Here's how the part is built. I have some questions about the finished solid (model axes, mm). Face numbers are marked on the shaded views. A direction names the side the tool comes from. Coordinates: 2 decimals unless noted, no trailing zeros. Use one line per item in the form item = value. Start each with the question number.
from build123d import *

# Parameters (mm, degrees)
SCHIZZO1_W                     = 23
SCHIZZO1_H                     = 23
ESTRUSIONE_ESTRUSIONE1_DEPTH   = 50
SCHIZZO3_R                     = 17
TAGLIO_ESTRUSIONE2_DEPTH       = 58.057295879
SCHIZZO4_R                     = 17
SCHIZZO4_R_2                   = 15
ESTRUSIONE_ESTRUSIONE2_DEPTH   = 23
ESTRUSIONE_ESTRUSIONE3_START   = -2
SCHIZZO6_R                     = 15
ESTRUSIONE_ESTRUSIONE3_DEPTH   = 2
ESTRUSIONE_ESTRUSIONE4_START   = 1
SCHIZZO11_R                    = 15
ESTRUSIONE_ESTRUSIONE4_DEPTH   = 1
SMUSSO2_SIZE                   = 2
SCHIZZO12_R                    = 2.5
TAGLIO_ESTRUSIONE6_DEPTH       = 85.53268453
SCHIZZO13_R                    = 4.75
TAGLIO_ESTRUSIONE7_DEPTH       = 2
SCHIZZO14_R                    = 1.5
TAGLIO_ESTRUSIONE9_DEPTH       = 85.53268453
TAGLIO_ESTRUSIONE11_DEPTH      = 85.53268453
TAGLIO_ESTRUSIONE12_REACH      = 85.286
TAGLIO_ESTRUSIONE12_END_RADIUS = 15
SCHIZZO18_R                    = 7.1
ESTRUSIONE_ESTRUSIONE5_REACH   = 87.292
SCHIZZO19_W                    = 4
SCHIZZO19_H                    = 3
SCHIZZO21_R                    = 5.5
ESTRUSIONE_ESTRUSIONE6_DEPTH   = 2
SCHIZZO20_R                    = 1.75
TAGLIO_ESTRUSIONE13_DEPTH      = 86.853216328
SMUSSO3_SIZE                   = 2
SMUSSO4_SIZE                   = 1
SMUSSO4_SIZE2                  = 3


with BuildPart() as part:
    # Schizzo1 → Estrusione-Estrusione1 (new body)
    with BuildSketch(Plane.XY):
        with Locations((-3.551080126, 2.313028552)):
            Rectangle(SCHIZZO1_W, SCHIZZO1_H)
    extrude(amount=ESTRUSIONE_ESTRUSIONE1_DEPTH)

    # Schizzo3 → Taglio-Estrusione2 (cut, through all)
    with BuildSketch(Plane(origin=(0, 13.813028552, 0), x_dir=(1, 0, 0), z_dir=(0, 1, 0))):
        with Locations((-3.551080126, -62.519984026)):
            Circle(SCHIZZO3_R)
    extrude(amount=-TAGLIO_ESTRUSIONE2_DEPTH, mode=Mode.SUBTRACT)

    # Schizzo4 → Estrusione-Estrusione2 (add, through all)
    with BuildSketch(Plane(origin=(0, 13.813028552, 0), x_dir=(1, 0, 0), z_dir=(0, 1, 0))):
        with Locations((-3.551080126, -62.519984026)):
            Circle(SCHIZZO4_R)
        with Locations(Location((-3.551080126, -62.519984026, 0), (0, 0, 180))):
            Circle(SCHIZZO4_R_2, mode=Mode.SUBTRACT)
    extrude(amount=-ESTRUSIONE_ESTRUSIONE2_DEPTH)

    # Schizzo6 → Estrusione-Estrusione3 (add)
    with BuildSketch(Plane.XZ.offset(9.186971448).offset(ESTRUSIONE_ESTRUSIONE3_START)):
        with Locations(Location((-3.551080126, 62.519984026, 0), (0, 0, 180))):
            Circle(SCHIZZO6_R)
    extrude(amount=ESTRUSIONE_ESTRUSIONE3_DEPTH)

    # Schizzo11 → Estrusione-Estrusione4 (add)
    with BuildSketch(Plane(origin=(0, -7.186971448, 0), x_dir=(1, 0, 0), z_dir=(0, 1, 0)).offset(ESTRUSIONE_ESTRUSIONE4_START)):
        with Locations(Location((-3.551080126, -62.519984026, 0), (0, 0, 180))):
            Circle(SCHIZZO11_R)
    extrude(amount=-ESTRUSIONE_ESTRUSIONE4_DEPTH)

    # Smusso2
    smusso2_edges = [part.edges().sort_by_distance(p)[0] for p in [
        (-3.551080126, -9.186971448, 79.519984026),
    ]]
    chamfer(smusso2_edges, length=SMUSSO2_SIZE)

    # Schizzo12 → Taglio-Estrusione6 (cut, through all)
    with BuildSketch(Plane(origin=(0, -6.186971448, 0), x_dir=(1, 0, 0), z_dir=(0, 1, 0))):
        with Locations(Location((-3.551080126, -62.519984026, 0), (0, 0, 270))):
            Circle(SCHIZZO12_R)
    extrude(amount=-TAGLIO_ESTRUSIONE6_DEPTH, mode=Mode.SUBTRACT)

    # Schizzo13 → Taglio-Estrusione7 (cut)
    with BuildSketch(Plane(origin=(0, -6.186971448, 0), x_dir=(1, 0, 0), z_dir=(0, 1, 0))):
        with Locations(Location((-3.551080126, -62.519984026, 0), (0, 0, 270))):
            Circle(SCHIZZO13_R)
    extrude(amount=-TAGLIO_ESTRUSIONE7_DEPTH, mode=Mode.SUBTRACT)

    # Schizzo14 → Taglio-Estrusione9 (cut, through all)
    with BuildSketch(Plane(origin=(0, -6.186971448, 0), x_dir=(1, 0, 0), z_dir=(0, 1, 0))):
        with Locations(Location((-9.808086042, -55.37156623, 0), (0, 0, 180))):
            Circle(SCHIZZO14_R)
        with Locations(Location((2.705925789, -69.668401821, 0), (0, 0, 180))):
            Circle(SCHIZZO14_R)
        with Locations(Location((-9.570800375, -67.789041638, 0), (0, 0, 180))):
            Circle(SCHIZZO14_R)
        with Locations(Location((2.468640122, -57.250926413, 0), (0, 0, 180))):
            Circle(SCHIZZO14_R)
    extrude(amount=-TAGLIO_ESTRUSIONE9_DEPTH, mode=Mode.SUBTRACT)

    # Schizzo17 → Taglio-Estrusione11 (cut, through all)
    with BuildSketch(Plane(origin=(0, -6.186971448, 0), x_dir=(1, 0, 0), z_dir=(0, 1, 0))):
        with BuildLine():
            Line((-5.034715393, -69.299017071), (-5.727078518, -73.947740907))
            ThreePointArc((-5.727078518, -73.947740907), (-3.551080126, -76.471825774), (-1.375081735, -73.947740907))
            Line((-1.375081735, -73.947740907), (-2.06744486, -69.299017071))
            ThreePointArc((-2.06744486, -69.299017071), (-3.551080126, -68.019984026), (-5.034715393, -69.299017071))
        make_face()
        with BuildLine():
            Line((3.227952919, -64.003619292), (7.876676755, -64.695982417))
            ThreePointArc((7.876676755, -64.695982417), (10.400761622, -62.519984026), (7.876676755, -60.343985634))
            Line((7.876676755, -60.343985634), (3.227952919, -61.036348759))
            ThreePointArc((3.227952919, -61.036348759), (1.948919874, -62.519984026), (3.227952919, -64.003619292))
        make_face()
        with BuildLine():
            Line((-10.330113172, -61.036348759), (-14.978837008, -60.343985634))
            ThreePointArc((-14.978837008, -60.343985634), (-17.502921875, -62.519984026), (-14.978837008, -64.695982417))
            Line((-14.978837008, -64.695982417), (-10.330113172, -64.003619292))
            ThreePointArc((-10.330113172, -64.003619292), (-9.051080126, -62.519984026), (-10.330113172, -61.036348759))
        make_face()
        with BuildLine():
            Line((-2.06744486, -55.74095098), (-1.375081735, -51.092227144))
            ThreePointArc((-1.375081735, -51.092227144), (-3.551080126, -48.568142277), (-5.727078518, -51.092227144))
            Line((-5.727078518, -51.092227144), (-5.034715393, -55.74095098))
            ThreePointArc((-5.034715393, -55.74095098), (-3.551080126, -57.019984026), (-2.06744486, -55.74095098))
        make_face()
    extrude(amount=-TAGLIO_ESTRUSIONE11_DEPTH, mode=Mode.SUBTRACT)

    # Taglio-Estrusione12: up to this cylinder (the profile starts outside it)
    taglio_estrusione12_end = Plane(origin=(-3.551080126, 2.313029, 62.519984026), z_dir=(0, 1, 0)) * Cylinder(TAGLIO_ESTRUSIONE12_END_RADIUS, 201.572, mode=Mode.PRIVATE)
    # Schizzo18 → Taglio-Estrusione12 (cut, up to the surface)
    with BuildSketch(Plane(origin=(0, 0, 0), x_dir=(-1, 0, 0), z_dir=(0, 0, -1)), mode=Mode.PRIVATE) as taglio_estrusione12_sk1:
        with Locations((3.551080126, 2.313028552)):
            Circle(SCHIZZO18_R)
    taglio_estrusione12_tool1 = extrude(taglio_estrusione12_sk1.sketch, amount=-TAGLIO_ESTRUSIONE12_REACH, mode=Mode.PRIVATE) - taglio_estrusione12_end
    add(taglio_estrusione12_tool1.solids().sort_by_distance((-3.55108, 2.313029, 0))[0], mode=Mode.SUBTRACT)

    # Schizzo19 → Estrusione-Estrusione5 (add, up to next)
    with BuildSketch(Plane(origin=(0, 13.813028552, 0), x_dir=(1, 0, 0), z_dir=(0, 1, 0)), mode=Mode.PRIVATE) as estrusione_estrusione5_sk1:
        with Locations((-3.551080126, -44.019984026)):
            Rectangle(SCHIZZO19_W, SCHIZZO19_H)
    estrusione_estrusione5_tool1 = extrude(estrusione_estrusione5_sk1.sketch, amount=-ESTRUSIONE_ESTRUSIONE5_REACH, mode=Mode.PRIVATE) - part.part
    add(estrusione_estrusione5_tool1.solids().sort_by_distance((-3.55108, 13.813029, 44.019984))[0])

    # Schizzo21 → Estrusione-Estrusione6 (add)
    with BuildSketch(Plane(origin=(0, 13.813028552, 0), x_dir=(1, 0, 0), z_dir=(0, 1, 0))):
        with Locations((-3.551080126, -9)):
            Circle(SCHIZZO21_R)
        with Locations((-3.551080126, -28)):
            Circle(SCHIZZO21_R)
    extrude(amount=ESTRUSIONE_ESTRUSIONE6_DEPTH)

    # Schizzo20 → Taglio-Estrusione13 (cut, through all)
    with BuildSketch(Plane(origin=(0, 15.813028552, 0), x_dir=(1, 0, 0), z_dir=(0, 1, 0))):
        with Locations(Location((-3.551080126, -9, 0), (0, 0, 180))):
            Circle(SCHIZZO20_R)
        with Locations(Location((-3.551080126, -28, 0), (0, 0, 180))):
            Circle(SCHIZZO20_R)
    extrude(amount=-TAGLIO_ESTRUSIONE13_DEPTH, mode=Mode.SUBTRACT)

    # Smusso3
    smusso3_edges = [part.edges().sort_by_distance(p)[0] for p in [
        (-9.051080126, 15.813028552, 9),
        (-9.051080126, 15.813028552, 28),
    ]]
    chamfer(smusso3_edges, length=SMUSSO3_SIZE - 0.0001)  # a hair under: the kernel refuses the full size

    # Smusso4
    smusso4_edges = [part.edges().sort_by_distance(p)[0] for p in [
        (3.548919874, 2.313028552, 0),
    ]]
    smusso4_side = [part.faces().sort_by_distance(p)[0] for p in [
        (-3.551080126, 13.487759433, 0),
    ]]
    chamfer(smusso4_edges, length=SMUSSO4_SIZE, length2=SMUSSO4_SIZE2, reference=smusso4_side[0])


solid = part.part
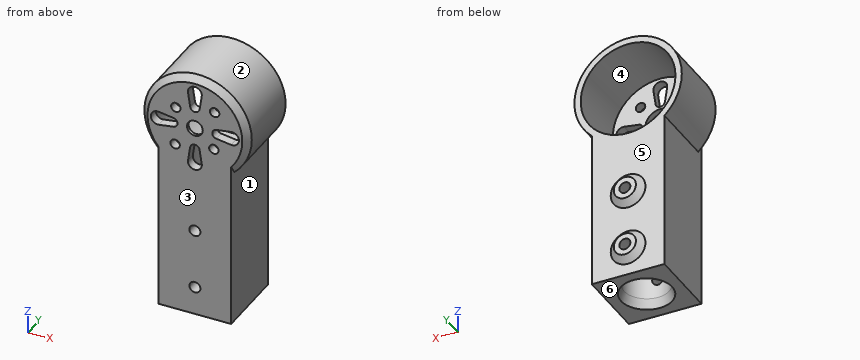
1) If we mould it in two halves opening along X, with no side actions, what happens to the marked faces 1, 2, 3 and 4? For each: pulls with the +X half, pulls with the -X half, needs draft (parallel to the pull), parting line crosses it, or undercut.
2) Which directions (+Z, -Z, +X, -X, +Y, -Y) give clear straight access to the entire face, cutting with the end or side of a thin tool? Please do the marked faces 5 and 6.
3) I need wall thicknesses on probe 1 along X at (y, z) = (3, 11.5); probe 2 along Z at (x, y) = (-14.5, 6); probe 3 along Y at (x, z) = (7.5, 20). Which ranges of each line are inside material? Lowest first, please. Write a range as [from, to].
4) For pin 1 (10 mm diameter, centred on x = 4.5, y = -6.5, fed in from +Z); pin 2 (7 mm diameter, centred on x = -3.55, z = 50.77, fed in from +Y); pin 3 (5 mm diameter, centred on y = 1, z = 25.5, fed in from -X); pin 4 (3 mm diameter, centred on x = -3.55, z = 62.52, fed in from +Y), each with a flat end and sliding along its axis, tell me the tip position at first contact or that it passes through.
From the geometry:
q1.face_1 = pulls with the +X half
q1.face_2 = parting line crosses it
q1.face_3 = needs draft
q1.face_4 = undercut
q2.face_5 = +Y
q2.face_6 = -Z, +X, -X, +Y, -Y
q3.probe_1 = [-15.05, -10.62], [3.52, 7.95]
q3.probe_2 = [0, 52.27], [72.77, 75.52]
q3.probe_3 = [-9.19, 13.81]
q4.pin_1 = 79.24
q4.pin_2 = 13.81
q4.pin_3 = -15.05
q4.pin_4 = through
